```python
from build123d import *

# Parameters (mm, degrees)
F2_R     = 3.81
F3_DEPTH = 9.525
F4_R     = 1.5875
F5_DEPTH = 12.7


with BuildPart() as f1:
    # F0 (on Front) → F1 (revolve)
    with BuildSketch(Plane.XZ):
        Polygon((0, 24.310512), (0, 0), (22.155415, 12.421659), (19.05, 17.960512), (6.35, 17.960512), (6.35, 24.310512), align=None)
    revolve(axis=Axis((0, 0, 12.155256), (0, 0, -1)))

    # F2 (on face) → F3 (cut)
    with BuildSketch(Plane.XY.offset(24.310512)):
        Circle(F2_R)
    extrude(amount=-F3_DEPTH, mode=Mode.SUBTRACT)

    # F4 (on Top) → F5 (cut)
    with BuildSketch(Plane.XY):
        Circle(F4_R)
    extrude(amount=F5_DEPTH, mode=Mode.SUBTRACT)


solid = f1.part
```
Input: part model. Units: mm. Frame: model coordinates. A direction names the side the tool comes from. Give positions to 0.01 mm unless a question says otherwise; leave off trailing zeros. Order: outer loops, then holes, each group sorted by start corner. A loop starts at its lowest first (then second) coordinate and runs counter-clockwise, first axis right, second up. Notation, with made-up numbers: (74.5, 59.5) -> (118.5, 59.5) arc R24 ccw to (118.5, 88.5) -> close; hole circle Ø10 at (-4.5, -33.75). An arc over 180 degrees is marked (long way). Write each question's results on one line, items separated by ' | '. Start each with the question number.
Item 1: Contact query for flat-ended pins moving along their axis: P1, Ø12, axis at y = -0.5, z = 21.5, coming from the +X side; P2, Ø4, axis at x = -1.5, z = 6, coming from the +Y side; P3, Ø1.5, axis at x = -5, z = 8, coming from the -Y side; P4, Ø1.5, axis at y = 11.5, z = 19.5, coming from the +X side. Output: stop coordinate, or through.
Item 2: Line query: line 1 (Y direction, x = 0, z = 20.5); line 2 (X direction, y = 1, z = 18); line 3 (Y direction, x = 0, z = 8.5). Output: solid intervals per line, ascending.
Item 3: Cut plane D-D on z = 17. Return the cut outline in (x, y).
Item 4: Set-up query: faces 4 (the flat face through (0, 0, 12.7)), 5 (the flat face through (0, 0, 14.786)). Return all of +Z, -Z, +X, -X, +Y, -Y with unobstructed straight access to the full face (end or side cutting, diameter ignored); none if empty.
Item 5: Mould query, pull axis X, two halves, no side actions, for faces 1 (the flat face through (3, 3, 24.311)), 2 (the conical face through (8.86, 17.034, 17.692)), 3 (the cylindrical face through (-0.34, -1.55, 6.71)). Classes: pulls with the +X half, pulls with the -X half, needs draft (parallel to the pull), parting line crosses it, or undercut.
Item 6: Cut plane C-C on z = 7.25. Return the cut outline in (x, y) (1 decimal).
Item 7: Cut plane A-A on y = 0. Return the cut outline in (x, z).
Established:
1) P1: x = 20.43 | P2: y = 14.2 | P3: y = -14.81 | P4: through
2) line 1: -6.35 to -3.81, 3.81 to 6.35 | line 2: -6.27 to -3.68, 3.68 to 6.27 | line 3: -15.16 to -1.59, 1.59 to 15.16
3) outline: circle Ø39.18 at (0, 0); hole circle Ø7.62 at (0, 0)
4) face 4: -Z | face 5: +Z
5) face 1: needs draft | face 2: parting line crosses it | face 3: undercut
6) outline: circle Ø25.9 at (0, 0); hole circle Ø3.2 at (0, 0)
7) outline: (-22.16, 12.42) -> (-1.59, 0.89) -> (-1.59, 12.7) -> (1.59, 12.7) -> (1.59, 0.89) -> (22.16, 12.42) -> (19.05, 17.96) -> (6.35, 17.96) -> (6.35, 24.31) -> (3.81, 24.31) -> (3.81, 14.79) -> (-3.81, 14.79) -> (-3.81, 24.31) -> (-6.35, 24.31) -> (-6.35, 17.96) -> (-19.05, 17.96) -> close
